from build123d import *

# Parameters (mm, degrees)
ESBO_O1_W                   = 230
ESBO_O1_H                   = 250
RESSALTO_EXTRUS_O1_DEPTH    = 6
ESBO_O2_R                   = 1.6
MOTOR_DEPTH                 = 6
ESBO_O4_R                   = 4.1
ESBO_O4_R_2                 = 1.6
GARRA_DEPTH                 = 10
ESBO_O7_R                   = 1.65
SENSORES_FRONTAIS_DEPTH     = 10
ESBO_O5_R                   = 1.6
ESBO_O5_R_2                 = 1.55
MAOS_FRANCESAS_DEPTH        = 10
ESPELHAR2_COPY_1_SKETCH_R   = 1.6
ESPELHAR2_COPY_1_DEPTH      = 6
ESPELHAR2_COPY_2_SKETCH_R   = 1.65
ESPELHAR2_COPY_2_DEPTH      = 10
ESPELHAR2_COPY_3_SKETCH_R   = 1.6
ESPELHAR2_COPY_3_SKETCH_R_2 = 1.55
ESPELHAR2_COPY_3_DEPTH      = 10
SENSORES_LATERAIS_DEPTH     = 10
FIOS_DEPTH                  = 10
ESBO_O10_R                  = 1.5
CORTE_EXTRUS_O7_DEPTH       = 10


with BuildPart() as part:
    # Esboço1 → Ressalto-extrusão1 (new body)
    with BuildSketch(Plane.XY):
        Rectangle(ESBO_O1_W, ESBO_O1_H)
    extrude(amount=RESSALTO_EXTRUS_O1_DEPTH)

    # Esboço2 → motor (cut)
    with BuildSketch(Plane.XY.offset(6)):
        with Locations((-60, 100)):
            Circle(ESBO_O2_R)
        with Locations((-30, 100)):
            Circle(ESBO_O2_R)
        with Locations((-30, 60)):
            Circle(ESBO_O2_R)
        with Locations((-60, 60)):
            Circle(ESBO_O2_R)
        Polygon((-75, 64), (-75, 54), (-115, 54), (-115, 106), (-75, 106), (-75, 96), (-10, 96), (-10, 64), align=None)
    motor = extrude(amount=-MOTOR_DEPTH, mode=Mode.SUBTRACT)

    # Esboço4 → garra (cut)
    with BuildSketch(Plane.XY.offset(6)):
        with Locations((-105, 35)):
            Circle(ESBO_O4_R)
        with Locations((-44.974586998, 39.2875295)):
            Circle(ESBO_O4_R_2)
        with Locations((-95.025413002, 35.7124705)):
            Circle(ESBO_O4_R_2)
        with Locations((-35, 40)):
            Circle(ESBO_O4_R)
        with Locations((-44.974586998, -39.2875295)):
            Circle(ESBO_O4_R_2)
        with Locations((-35, -40)):
            Circle(ESBO_O4_R)
        with Locations((-95.025413002, -35.7124705)):
            Circle(ESBO_O4_R_2)
        with Locations((-105, -35)):
            Circle(ESBO_O4_R)
        with Locations((-75, 35)):
            Circle(ESBO_O4_R_2)
        with Locations((-75, -35)):
            Circle(ESBO_O4_R_2)
    extrude(amount=-GARRA_DEPTH, mode=Mode.SUBTRACT)

    # Esboço7 → sensores frontais (cut)
    with BuildSketch(Plane.XY.offset(6)):
        with Locations((-105, 111)):
            Circle(ESBO_O7_R)
        with Locations((-90, 111)):
            Circle(ESBO_O7_R)
        with BuildLine():
            Line((-15, 111.35), (-55, 111.35))
            ThreePointArc((-55, 111.35), (-56.65, 113), (-55, 114.65))
            Line((-55, 114.65), (-15, 114.65))
            ThreePointArc((-15, 114.65), (-13.35, 113), (-15, 111.35))
        make_face()
    sensores_frontais = extrude(amount=-SENSORES_FRONTAIS_DEPTH, mode=Mode.SUBTRACT)

    # Esboço5 → maos francesas (cut)
    with BuildSketch(Plane(origin=(0, 0, 0), x_dir=(-1, 0, 0), z_dir=(0, 0, -1))):
        with Locations((70, 109)):
            Circle(ESBO_O5_R)
        with Locations((-102, 47.5)):
            Circle(ESBO_O5_R_2)
        with Locations((-103, 120)):
            Circle(ESBO_O5_R_2)
        with Locations((11, 50)):
            Circle(ESBO_O5_R)
        Circle(ESBO_O5_R_2)
        with Locations((-11, 50)):
            Circle(ESBO_O5_R)
        with Locations((-11, -50)):
            Circle(ESBO_O5_R)
        with Locations((11, -50)):
            Circle(ESBO_O5_R)
    maos_francesas = extrude(amount=-MAOS_FRANCESAS_DEPTH, mode=Mode.SUBTRACT)

    # Espelhar1: motor, sensores frontais, maos francesas across plane
    add(motor.mirror(Plane(origin=(0, 0, 0), x_dir=(0, 0, 1), z_dir=(1, 0, 0))), mode=Mode.SUBTRACT)
    add(sensores_frontais.mirror(Plane(origin=(0, 0, 0), x_dir=(0, 0, 1), z_dir=(1, 0, 0))), mode=Mode.SUBTRACT)
    add(maos_francesas.mirror(Plane(origin=(0, 0, 0), x_dir=(0, 0, 1), z_dir=(1, 0, 0))), mode=Mode.SUBTRACT)

    # Espelhar2: motor, sensores frontais, maos francesas across plane
    add(motor.mirror(Plane.ZX), mode=Mode.SUBTRACT)
    add(sensores_frontais.mirror(Plane.ZX), mode=Mode.SUBTRACT)
    add(maos_francesas.mirror(Plane.ZX), mode=Mode.SUBTRACT)

    # Espelhar2 copy 1 sketch → Espelhar2 copy 1 (cut)
    with BuildSketch(Plane(origin=(0, 0, 6), x_dir=(-1, 0, 0), z_dir=(0, 0, 1))):
        with Locations((-60, 100)):
            Circle(ESPELHAR2_COPY_1_SKETCH_R)
        with Locations((-30, 100)):
            Circle(ESPELHAR2_COPY_1_SKETCH_R)
        with Locations((-30, 60)):
            Circle(ESPELHAR2_COPY_1_SKETCH_R)
        with Locations((-60, 60)):
            Circle(ESPELHAR2_COPY_1_SKETCH_R)
        Polygon((-75, 64), (-75, 54), (-115, 54), (-115, 106), (-75, 106), (-75, 96), (-10, 96), (-10, 64), align=None)
    extrude(amount=-ESPELHAR2_COPY_1_DEPTH, mode=Mode.SUBTRACT)

    # Espelhar2 copy 2 sketch → Espelhar2 copy 2 (cut)
    with BuildSketch(Plane(origin=(0, 0, 6), x_dir=(-1, 0, 0), z_dir=(0, 0, 1))):
        with Locations((-105, 111)):
            Circle(ESPELHAR2_COPY_2_SKETCH_R)
        with Locations((-90, 111)):
            Circle(ESPELHAR2_COPY_2_SKETCH_R)
        with BuildLine():
            Line((-15, 111.35), (-55, 111.35))
            ThreePointArc((-55, 111.35), (-56.65, 113), (-55, 114.65))
            Line((-55, 114.65), (-15, 114.65))
            ThreePointArc((-15, 114.65), (-13.35, 113), (-15, 111.35))
        make_face()
    extrude(amount=-ESPELHAR2_COPY_2_DEPTH, mode=Mode.SUBTRACT)

    # Espelhar2 copy 3 sketch → Espelhar2 copy 3 (cut)
    with BuildSketch(Plane(origin=(0, 0, 0), x_dir=(1, 0, 0), z_dir=(0, 0, -1))):
        with Locations((70, 109)):
            Circle(ESPELHAR2_COPY_3_SKETCH_R)
        with Locations((-102, 47.5)):
            Circle(ESPELHAR2_COPY_3_SKETCH_R_2)
        with Locations((-103, 120)):
            Circle(ESPELHAR2_COPY_3_SKETCH_R_2)
        with Locations((11, 50)):
            Circle(ESPELHAR2_COPY_3_SKETCH_R)
        Circle(ESPELHAR2_COPY_3_SKETCH_R_2)
        with Locations((-11, 50)):
            Circle(ESPELHAR2_COPY_3_SKETCH_R)
        with Locations((-11, -50)):
            Circle(ESPELHAR2_COPY_3_SKETCH_R)
        with Locations((11, -50)):
            Circle(ESPELHAR2_COPY_3_SKETCH_R)
    extrude(amount=-ESPELHAR2_COPY_3_DEPTH, mode=Mode.SUBTRACT)

    # Esboço8 → Sensores laterais (cut)
    with BuildSketch(Plane.XY.offset(6)):
        with BuildLine():
            Line((-98.65, -21), (-98.65, 21))
            ThreePointArc((-98.65, 21), (-97, 22.65), (-95.35, 21))
            Line((-95.35, 21), (-95.35, -21))
            ThreePointArc((-95.35, -21), (-97, -22.65), (-98.65, -21))
        make_face()
        with BuildLine():
            Line((98.65, -21), (98.65, 21))
            ThreePointArc((98.65, 21), (97, 22.65), (95.35, 21))
            Line((95.35, 21), (95.35, -21))
            ThreePointArc((95.35, -21), (97, -22.65), (98.65, -21))
        make_face()
    extrude(amount=-SENSORES_LATERAIS_DEPTH, mode=Mode.SUBTRACT)

    # Esboço9 → Fios (cut)
    with BuildSketch(Plane(origin=(0, 0, 0), x_dir=(-1, 0, 0), z_dir=(0, 0, -1))):
        with BuildLine():
            Line((-35, 50), (-25, 50))
            ThreePointArc((-25, 50), (-20, 45), (-25, 40))
            Line((-25, 40), (-35, 40))
            ThreePointArc((-35, 40), (-40, 45), (-35, 50))
        make_face()
        with BuildLine():
            Line((-35, -50), (-25, -50))
            ThreePointArc((-25, -50), (-20, -45), (-25, -40))
            Line((-25, -40), (-35, -40))
            ThreePointArc((-35, -40), (-40, -45), (-35, -50))
        make_face()
    extrude(amount=-FIOS_DEPTH, mode=Mode.SUBTRACT)

    # Esboço10 → Corte-extrusão7 (cut)
    with BuildSketch(Plane(origin=(0, 0, 0), x_dir=(-1, 0, 0), z_dir=(0, 0, -1))):
        with Locations((-95, 24.686677652)):
            Circle(ESBO_O10_R)
        with Locations((-93.76, -23.483322348)):
            Circle(ESBO_O10_R)
        with Locations((-11.46, -23.483322348)):
            Circle(ESBO_O10_R)
    extrude(amount=-CORTE_EXTRUS_O7_DEPTH, mode=Mode.SUBTRACT)


solid = part.part
Geometry check sheet. Reference: the model listing, model coordinates, mm. A direction names the side the tool comes from. Coordinates: 2 decimals unless noted, no trailing zeros. Order: outer loops, then holes, each group sorted by start corner. A loop starts at its lowest first (then second) coordinate and runs counter-clockwise, first axis right, second up. Notation, with made-up numbers: (12, 23) - (38, 23) arc R22 cw to (38, 38) - close; hole circle Ø1 at (4, -10.5). An arc over 180 degrees is marked (long way). One line per item, written item: value.
(1) Sectioned sample at C-C (z = 2.2). Count the separate pieces of the cut face and the enclosed holes in it, and give its area (3 significant figures).
Data:
separate pieces: 1
enclosed holes: 62
area: 39,000 mm^2
(2) Sectioned sample at A-A (y = 18). Enter the section's corners in (x, z).
Data:
outline: (-115, 0) - (-98.65, 0) - (-98.65, 6) - (-115, 6) - close; (-95.35, 0) - (95.35, 0) - (95.35, 6) - (-95.35, 6) - close; (98.65, 0) - (115, 0) - (115, 6) - (98.65, 6) - close
(3) Thickness scan on probe 1 along Y at (x, z) = (41.5, 4.45); probe 2 along Y at (x, z) = (-13, 4.5); probe 3 along X at (y, z) = (120, 1.85). Record the ranges inside material, lowest first. Write a range as from..to.
Data:
probe 1: y = -125..-114.65, -111.35..-96, -64..64, 96..111.35, 114.65..125
probe 2: y = -125..-96, -64..64, 96..125
probe 3: x = -115..-104.55, -101.45..101.45, 104.55..115
(4) Sectioned sample at B-B (y = 68.5). Enter the section's corners in (x, z), and give its area (3 significant figures).
Data:
outline: (-10, 0) - (10, 0) - (10, 6) - (-10, 6) - close
area: 120 mm^2
(5) Depth check by flat-ended pin: pin 1 Ø3 at (y, z) = (-103, 3) entering from +X. Enter the tip coordinate at first touch or a pass-through.
Data:
pin 1: stops at x = 75
(6) Release check for a two-part mould opening along Y. For faces 1 (the face through (115, -1, 3)), 2 (the face through (10, -80, 3)) record: +Y half, -Y half, draft (parallel to the pull), parting line (faces both ways), or undercut.
Data:
face 1: draft
face 2: undercut
(7) Access from +Z, -Z, +X, -X, +Y, -Y to the whole of each face (thin tool, end or side, straight path). Record for faces 3 (the face through (42, -64, 3)), 4 (the face through (-35, -114.65, 3)), 5 (the face through (-2, 2, 6)), 6 (the face through (-75, 101, 3)).
Data:
face 3: +Z, -Z, +X
face 4: +Z, -Z
face 5: +Z, +X, -X, +Y, -Y
face 6: +Z, -Z, -X
